Here's how the part is built. I have some questions about the finished solid (model axes, mm). A direction names the side the tool comes from. Round coordinates to 2 decimals unless told otherwise and drop trailing zeros. Order: outer loops, then holes, each group sorted by start corner. A loop starts at its lowest first (then second) coordinate and runs counter-clockwise, first axis right, second up. Notation, with made-up numbers: (24, 37.25) - (60, 37.25) arc R28 ccw to (60, 57.25) - close; hole circle Ø8 at (30, -31). An arc over 180 degrees is marked (long way). Answer as a JSON object with one key per item and string values.
```python
from build123d import *

# Parameters (mm, degrees)
SKETCH1_R           = 5.5
HANDLE_DEPTH        = 20
SKETCH2_R           = 5
SKETCH2_R_2         = 4
SLEEVE_DEPTH        = 7
SKETCH3_R           = 0.75
CENTRE_PIN_DEPTH    = 7
SKETCH4_R           = 3.5
STRAIN_RELIEF_DEPTH = 10
LEAD_PROFILE_R      = 2.5


with BuildPart() as part:
    # Sketch1 → Handle (new body)
    with BuildSketch(Plane(origin=(0, 0, 0), x_dir=(1, 0, 0), z_dir=(0, 1, 0))):
        with Locations(Location((0, 0, 0), (0, 0, 270))):
            Circle(SKETCH1_R)
    extrude(amount=-HANDLE_DEPTH)

    # Sketch2 → Sleeve (add)
    with BuildSketch(Plane(origin=(0, 0, 0), x_dir=(1, 0, 0), z_dir=(0, 1, 0))):
        with Locations(Location((0, 0, 0), (0, 0, 270))):
            Circle(SKETCH2_R)
        with Locations(Location((0, 0, 0), (0, 0, 270))):
            Circle(SKETCH2_R_2, mode=Mode.SUBTRACT)
    extrude(amount=SLEEVE_DEPTH)

    # Sketch3 → Centre_pin (add)
    with BuildSketch(Plane(origin=(0, 0, 0), x_dir=(1, 0, 0), z_dir=(0, 1, 0))):
        with Locations(Location((0, 0, 0), (0, 0, 270))):
            Circle(SKETCH3_R)
    extrude(amount=CENTRE_PIN_DEPTH)

    # Sketch4 → Strain_relief (add)
    with BuildSketch(Plane(origin=(0, -20, 0), x_dir=(1, 0, 0), z_dir=(0, 1, 0))):
        with Locations(Location((0, 0, 0), (0, 0, 270))):
            Circle(SKETCH4_R)
    extrude(amount=-STRAIN_RELIEF_DEPTH)

    # Lead: sweep along a path in Sketch5
    with BuildLine(Plane(origin=(0, 0, 0), x_dir=(0, 0, -1), z_dir=(1, 0, 0))) as lead_path:
        Line((0, -30), (0, -35))
        ThreePointArc((0, -35), (5.857864376, -49.142135624), (20, -55))
        Line((20, -55), (52.7, -55))
        ThreePointArc((52.7, -55), (63.306601718, -59.393398282), (67.7, -70))
        Line((67.7, -70), (67.7, -110))
    # Lead profile (on start of the path) → Lead (sweep)
    with BuildSketch(Plane(origin=(0, -30, 0), x_dir=(0, 0, -1), z_dir=(0, -1, 0))):
        Circle(LEAD_PROFILE_R)
    sweep(path=lead_path.line)


solid = part.part
```
1. If I drill on L1, parallel to X at y = 4, z = 0; L2, parallel to Y at x = -0.5, z = -62; L3, parallel to Z at x = 2.5, y = -18.5, over which ranges is the centre line in solid material (lowest first)? Write a range as [from, to].
Responses:
{"L1": "[-5, -4], [-0.75, 0.75], [4, 5]", "L2": "[-61.57, -55.24]", "L3": "[-4.9, 4.9]"}
2. Imagine slicing it at A-A (y = -72.5). List the corners of the cut face in (x, z) for me.
Responses:
{"outline": "circle Ø5 at (0, -67.7)"}
3. Thinking about a two-plate mould opening in Y: for faces 1 (the face through (-4.88, 3.45, -1.08)), 2 (the face through (-2.44, -32.53, 0.54)), 3 (the face through (-0.96, -52.69, -36.58)), which applies, pulls with the +Y half, pulls with the -Y half, needs draft (parallel to the pull), parting line crosses it, or undercut?
Responses:
{"face 1": "needs draft", "face 2": "undercut", "face 3": "parting line crosses it"}
4. For faces 4 (the face through (-4.9, 0, 1.6)), 5 (the face through (0.1, -90.3, -65.2)), 6 (the face through (0, -20, 4)), which set-ups out of +Z, -Z, +X, -X, +Y, -Y let a thin tool reach every point of the face, with its end or its side?
Responses:
{"face 4": "+Y", "face 5": "-Y", "face 6": "none"}
5. Imagine slicing it at B-B (z = -48). List the corners of the cut face in (x, y) for me.
Responses:
{"outline": "circle Ø5 at (0, -55)"}
6. For P1, Ø3.5, axis at x = 0.5, z = 1.5, coming from the -Y side; P2, Ø8, axis at y = -49, z = -37, coming from the +X side; P3, Ø3, axis at x = 2, z = -39.5, coming from the +Y side, each with a flat end and sliding along its axis, tell me the tip position at first contact or that it passes through.
Responses:
{"P1": "y = -45.72", "P2": "x = 1.5", "P3": "y = -52.55"}
